Autodesk Inventor part; units mm, degrees
ref_plane "YZ Plane" through (0, 0, 0) normal (1, 0, 0) x (0, 1, 0)
ref_plane "XZ Plane" through (0, 0, 0) normal (0, 1, 0) x (-1, 0, 0)
ref_plane "XY Plane" through (0, 0, 0) normal (0, 0, 1) x (1, 0, 0)
sketch "草图1" plane through (0, 0, 0) normal (0, 0, 1) x (1, 0, 0)
  circle A0 centre (0, 0) radius 5
  dimension "d0" = 10
extrude "拉伸1" add sketch "草图1" along normal blind 1
sketch "草图2" plane through (0, 0, 1) normal (0, 0, 1) x (1, 0, 0)
  line L0 (2.0207, -3.5) -> (-2.0207, -3.5)
  line L1 (-2.0207, -3.5) -> (-4.0415, 0)
  line L2 (-4.0415, 0) -> (-2.0207, 3.5)
  line L3 (-2.0207, 3.5) -> (2.0207, 3.5)
  line L4 (2.0207, 3.5) -> (4.0415, 0)
  line L5 (4.0415, 0) -> (2.0207, -3.5)
  line L6 (0, 0) -> (0, 1.4053)
  circle A0 centre (0, 0) radius 5
  point P0 (0, 3.5)
  dimension "d3" = 1.4053
  dimension "d4" = 3.5
extrude "拉伸2" add sketch "草图2" along normal blind 4 contours L0 L1 L2 L3 L4 L5
fillet "圆角1" radius 0.5 13 edges at (-5, 0, 1) (2.0207, 3.5, 3) (0, 3.5, 5) (-2.0207, 3.5, 3) (-3.0311, 1.75, 5) (-4.0415, 0, 3) (-3.0311, -1.75, 5) (-2.0207, -3.5, 3) (0, -3.5, 5) (2.0207, -3.5, 3) (3.0311, -1.75, 5) (4.0415, 0, 3) (3.0311, 1.75, 5)
sketch "草图3" plane through (0, 0, 0) normal (0, 0, -1) x (-1, 0, 0)
  circle A0 centre (0, 0) radius 2.5
  dimension "d8" = 5
extrude "拉伸3" add sketch "草图3" along normal blind 28
thread "螺纹1"
chamfer "倒角1" distance 0.25 angle 45 1 edges at (2.5, 0, -28)
properties part number "主动轮护盖固定螺丝"
Geometry: final body of the model. Coordinates: model frame, mm. A direction names the side the tool comes from. Give positions to 0.01 mm unless a question says otherwise; leave off trailing zeros. Write each loop counter-clockwise with the first axis right and the second up, starting at its lowest first coordinate (ties: lowest second). Pieces come first, ordered by that corner, then holes.
1. Section query B-B, the plane z = -17.5. Return loops of the section in (x, y).
2. Section query A-A, the plane x = 0. Return loops of the section in (y, z).
3. Pin query (flat end, axial travel): P1, Ø4, axis at x = -4, z = -11, coming from the +Y side; P2, Ø1, axis at x = 0.5, z = 2.5, coming from the -Y side; P3, Ø1.5, axis at x = -2, z = 1, coming from the -Y side. Return the tip coordinate at first contact, or that it passes through.
4. Line query: probe 1 along Z at (x, y) = (2.5, -3.5); probe 2 along Y at (x, z) = (-1.25, -16.5); probe 3 along X at (y, z) = (1.5, -10.5). Output: solid intervals per line, ascending.
5. Reachability of faces 1 (the cylindrical face through (0.54, 2.44, -13.68)), 2 (the flat face through (3, 1.8, 2.7)), 3 (the flat face through (-3, -1.8, 2.7)), 4 (the flat face through (0, -4, 1)) from +Z, -Z, +X, -X, +Y, -Y: full face, straight path, thin tool, end or side. Return the list, or none.
Computed:
1. outline: circle Ø5 at (0, 0)
2. outline: (-5, 0) - (-2.5, 0) - (-2.5, -27.75) - (-2.25, -28) - (2.25, -28) - (2.5, -27.75) - (2.5, 0) - (5, 0) - (5, 0.5) arc R0.5 ccw to (4.5, 1) - (3.5, 1) - (3.5, 4.5) arc R0.5 ccw to (3, 5) - (-3, 5) arc R0.5 ccw to (-3.5, 4.5) - (-3.5, 1) - (-4.5, 1) arc R0.5 ccw to (-5, 0.5) - close
3. P1: stops at y = 1.5
3. P2: stops at y = -3.5
3. P3: stops at y = -4.8
4. probe 1: z = 0 to 1
4. probe 2: y = -2.17 to 2.17
4. probe 3: x = -2 to 2
5. face 1: -Z
5. face 2: +Z, +X, +Y
5. face 3: +Z, -X, -Y
5. face 4: +Z
